Check sheet for the modelled part. Datum: model origin and axes. Units: mm. A direction names the side the tool comes from. Coordinates: 2 decimals unless noted, no trailing zeros. Write each loop counter-clockwise with the first axis right and the second up, starting at its lowest first coordinate (ties: lowest second). Pieces come first, ordered by that corner, then holes. Notation, with made-up numbers: (-17.75, 8) - (15.25, 8) arc R4 cw to (15.25, 14) - close; hole circle Ø2 at (-32.75, 17). An arc over 180 degrees is marked (long way). Write each question's results on one line, items separated by ' | '.
from build123d import *

# Parameters (mm, degrees)
SKETCH_1_W          = 48
SKETCH_1_H          = 15
EXTRUDE_1_DEPTH     = 3
SKETCH_2_W          = 3
SKETCH_2_H          = 15
EXTRUDE_2_DEPTH     = 25
SKETCH_3_W          = 15
SKETCH_3_H          = 3
EXTRUDE_3_DEPTH     = 8
SKETCH_4_R          = 2.1
CUT_EXTRUDE_3_DEPTH = 100


with BuildPart() as part:
    # 草图1 → 凸台-拉伸1 (new body)
    with BuildSketch(Plane(origin=(0, 0, 0), x_dir=(1, 0, 0), z_dir=(0, 1, 0))):
        Rectangle(SKETCH_1_W, SKETCH_1_H)
    extrude(amount=EXTRUDE_1_DEPTH)

    # 草图2 → 凸台-拉伸2 (add)
    with BuildSketch(Plane(origin=(0, 0, 0), x_dir=(1, 0, 0), z_dir=(0, 1, 0))):
        with Locations((25.5, 0)):
            Rectangle(SKETCH_2_W, SKETCH_2_H)
        with Locations((-25.5, 0)):
            Rectangle(SKETCH_2_W, SKETCH_2_H)
    extrude(amount=EXTRUDE_2_DEPTH)

    # 草图3 → 凸台-拉伸3 (add)
    with BuildSketch(Plane(origin=(27, 0, 0), x_dir=(0, 0, -1), z_dir=(1, 0, 0))):
        with Locations((0, 23.5)):
            Rectangle(SKETCH_3_W, SKETCH_3_H)
    extrude_3 = extrude(amount=EXTRUDE_3_DEPTH)

    # 镜向1: 凸台-拉伸3 across plane
    add(extrude_3.mirror(Plane(origin=(0, 0, 0), x_dir=(0, 0, 1), z_dir=(1, 0, 0))))

    # 草图4 → 切除-拉伸3 (cut)
    with BuildSketch(Plane(origin=(0, 0, 0), x_dir=(1, 0, 0), z_dir=(0, 1, 0))):
        with Locations(Location((-31, 0, 0), (0, 0, 90))):
            Circle(SKETCH_4_R)
    cut_extrude_3 = extrude(amount=CUT_EXTRUDE_3_DEPTH, mode=Mode.SUBTRACT)

    # 镜向2: 切除-拉伸3 across plane
    add(cut_extrude_3.mirror(Plane(origin=(0, 0, 0), x_dir=(0, 0, 1), z_dir=(1, 0, 0))), mode=Mode.SUBTRACT)


solid = part.part
1. Access from +Z, -Z, +X, -X, +Y, -Y to the whole of each face (thin tool, end or side, straight path). Record for faces 5 (the flat face through (-27, 11, 0)), 6 (the flat face through (33, 22, 2)), 7 (the flat face through (24, 14, 0)).
Values follow:
face 5: +Z, -Z, -X, -Y | face 6: +Z, -Z, +X, -Y | face 7: +Z, -Z, +Y
2. Go/stop test with flat-tipped pins: pin 1 (8 mm diameter, centred on y = 5, z = -1.5, fed in from +X); pin 2 (5.5 mm diameter, centred on x = 31, z = 0, fed in from -Y); pin 3 (7.5 mm diameter, centred on y = 14, z = -3, fed in from -X). Record where each tip stops, or that it passes through.
Values follow:
pin 1: stops at x = 27 | pin 2: stops at y = 22 | pin 3: stops at x = -27
3. Sectioned sample at C-C (z = 0). Record the cut outline in (x, y), then the cut area to 3 significant figures.
Values follow:
outline: (-35, 22) - (-33.1, 22) - (-33.1, 25) - (-35, 25) - close; (-28.9, 22) - (-27, 22) - (-27, 0) - (27, 0) - (27, 22) - (28.9, 22) - (28.9, 25) - (24, 25) - (24, 3) - (-24, 3) - (-24, 25) - (-28.9, 25) - close; (33.1, 22) - (35, 22) - (35, 25) - (33.1, 25) - close | area: 317 mm^2
4. Draft check along Z on faces 1 (the flat face through (3, 2, -7.5)), 2 (the cylindrical face through (-28.95, 23.48, 0.46)), 3 (the flat face through (3, 2, 7.5)), 4 (the flat face through (-35, 24, 0)). Enter one of: pulls with the +Z half, pulls with the -Z half, needs draft (parallel to the pull), parting line crosses it, or undercut.
Values follow:
face 1: pulls with the -Z half | face 2: undercut | face 3: pulls with the +Z half | face 4: needs draft
5. Sectioned sample at B-B (x = -31). Record the cut outline in (y, z), then the cut area to 3 significant figures.
Values follow:
outline: (22, -7.5) - (25, -7.5) - (25, -2.1) - (22, -2.1) - close; (22, 2.1) - (25, 2.1) - (25, 7.5) - (22, 7.5) - close | area: 32.4 mm^2
6. Material ranges on L1, parallel to X at y = 23.35, z = 0; L2, parallel to X at y = 23.5, z = -3.5; L3, parallel to X at y = 6.5, z = 1, recorded low to high. Write a range as [from, to].
Values follow:
L1: x = [-35, -33.1], [-28.9, -24], [24, 28.9], [33.1, 35] | L2: x = [-35, -24], [24, 35] | L3: x = [-27, -24], [24, 27]
7. Sectioned sample at A-A (y = 7.5). Record the cut outline in (x, z).
Values follow:
outline: (-27, -7.5) - (-24, -7.5) - (-24, 7.5) - (-27, 7.5) - close; (24, -7.5) - (27, -7.5) - (27, 7.5) - (24, 7.5) - close
8. Sectioned sample at D-D (z = 6.5). Record the cut outline in (x, y).
Values follow:
outline: (-35, 22) - (-27, 22) - (-27, 0) - (27, 0) - (27, 22) - (35, 22) - (35, 25) - (24, 25) - (24, 3) - (-24, 3) - (-24, 25) - (-35, 25) - close
